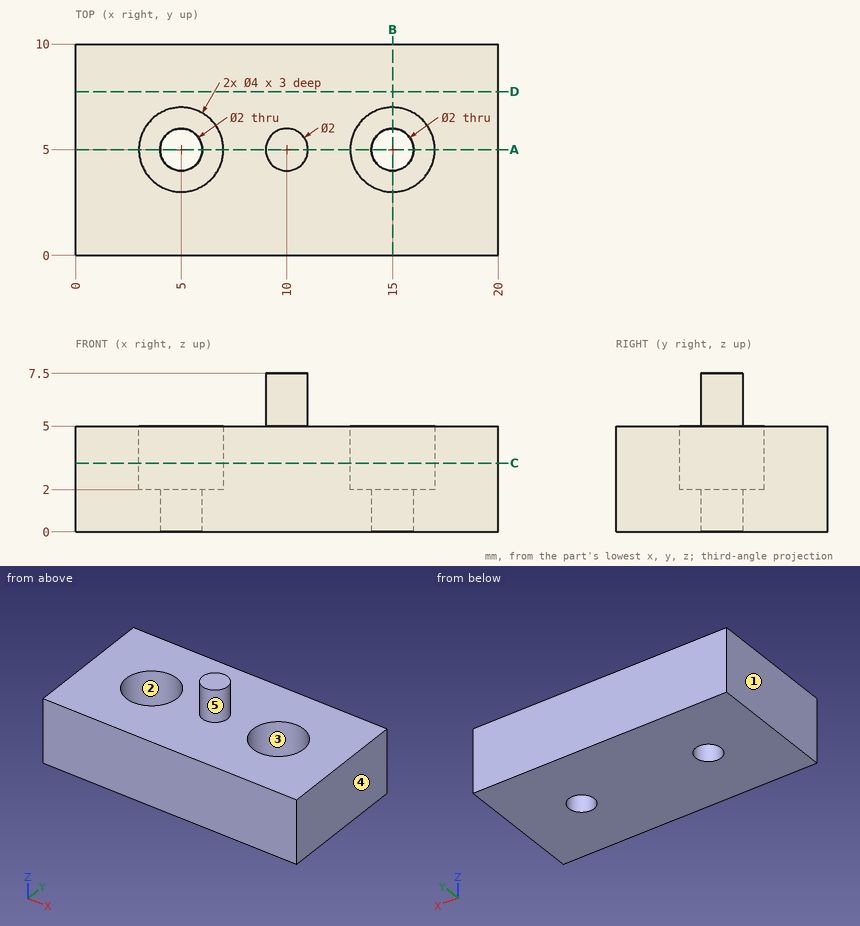
The drawing under review shows one solid part. Ordinate dimensions are in mm from its lowest x, y, z. A direction names the side the tool comes from. Give positions to 0.01 mm unless a question says otherwise; leave off trailing zeros. Write each loop counter-clockwise with the first axis right and the second up, starting at its lowest first coordinate (ties: lowest second). Pieces come first, ordered by that corner, then holes. Notation, with made-up numbers: (28.5, -13) -> (42.5, -13) arc R24 ccw to (42.5, 8) -> close; hole circle Ø4 at (-27, 72). An arc over 180 degrees is marked (long way). Put each result on its own line as item: value.
(1) We need section B-B, the plane x = 15. Give the boundary of the cut face in (y, z).
Results are:
outline: (0, 0) -> (4, 0) -> (4, 2) -> (3, 2) -> (3, 5) -> (0, 5) -> close; (6, 0) -> (10, 0) -> (10, 5) -> (7, 5) -> (7, 2) -> (6, 2) -> close
(2) The part is to be moulded in two halves that separate along Y. For the marked faces 3, 4 and 5, say which applies: pulls with the +Y half, pulls with the -Y half, needs draft (parallel to the pull), parting line crosses it, or undercut.
Results are:
face 3: undercut
face 4: needs draft
face 5: parting line crosses it
(3) For pin 1 Ø3 at (y, z) = (8.5, 5.5) entering from +X; pin 2 Ø4.5 at (x, y) = (14, 5) entering from +Z, all flat-tipped, find the tip position at first contact; note any pin that passes through.
Results are:
pin 1: x = 20
pin 2: z = 5
(4) We need section A-A, the plane y = 5. Give the boundary of the cut face in (x, z), and give its area (3 significant figures).
Results are:
outline: (0, 0) -> (4, 0) -> (4, 2) -> (3, 2) -> (3, 5) -> (0, 5) -> close; (6, 0) -> (14, 0) -> (14, 2) -> (13, 2) -> (13, 5) -> (11, 5) -> (11, 7.5) -> (9, 7.5) -> (9, 5) -> (7, 5) -> (7, 2) -> (6, 2) -> close; (16, 0) -> (20, 0) -> (20, 5) -> (17, 5) -> (17, 2) -> (16, 2) -> close
area: 73.0 mm²
(5) We need section D-D, the plane y = 7.75. Give the boundary of the cut face in (x, z), and give its area (3 significant figures).
Results are:
outline: (0, 0) -> (20, 0) -> (20, 5) -> (0, 5) -> close
area: 100 mm²
(6) To check wall thickness, follow probe 1 along X at (y, z) = (5, 0.85); probe 2 along Y at (x, z) = (5, 0.65); probe 3 along Y at (x, z) = (5, 4). State the ranges of each line that lie inside material, in increasing order. Write a range as from..to.
Results are:
probe 1: 0..4, 6..14, 16..20
probe 2: 0..4, 6..10
probe 3: 0..3, 7..10
(7) Tool access review of the marked faces 1 and 2: name each direction out of +Z, -Z, +X, -X, +Y, -Y from which nothing blocks a thin tool from reaching the whole face with its end or side.
Results are:
face 1: +Z, -Z, -X, +Y, -Y
face 2: +Z
(8) We need section C-C, the plane z = 3.25. Give the boundary of the cut face in (x, y), and give its area (3 significant figures).
Results are:
outline: (0, 0) -> (20, 0) -> (20, 10) -> (0, 10) -> close; hole circle Ø4 at (5, 5); hole circle Ø4 at (15, 5)
area: 175 mm²
